```python
from build123d import *

# Parameters (mm, degrees)
SKETCH1_W           = 66.5
SKETCH1_H           = 36
SKETCH1_W_2         = 60.5
SKETCH1_H_2         = 30
BOSS_EXTRUDE1_DEPTH = 71
SKETCH1_3_W         = 66.5
SKETCH1_3_H         = 36
SKETCH1_3_W_2       = 60.5
SKETCH1_3_H_2       = 30
BOSS_EXTRUDE2_DEPTH = 3
CUT_EXTRUDE1_REACH  = 88.27
SKETCH2_W           = 15
SKETCH2_H           = 10
SKETCH4_W           = 1
SKETCH4_H           = 2
BOSS_EXTRUDE4_DEPTH = 15
CHAMFER1_SIZE       = 1
CUT_EXTRUDE2_DEPTH  = 1


with BuildPart() as part:
    # Sketch1 → Boss-Extrude1 (new body)
    with BuildSketch(Plane(origin=(0, 0, 0), x_dir=(1, 0, 0), z_dir=(0, 1, 0))):
        Rectangle(SKETCH1_W, SKETCH1_H)
        Rectangle(SKETCH1_W_2, SKETCH1_H_2, mode=Mode.SUBTRACT)
    extrude(amount=BOSS_EXTRUDE1_DEPTH)

    # Sketch1<3> → Boss-Extrude2 (add)
    with BuildSketch(Plane(origin=(0, 0, 0), x_dir=(1, 0, 0), z_dir=(0, 1, 0))):
        Rectangle(SKETCH1_3_W, SKETCH1_3_H)
        Rectangle(SKETCH1_3_W_2, SKETCH1_3_H_2, mode=Mode.SUBTRACT)
        Rectangle(SKETCH1_3_W_2, SKETCH1_3_H_2)
    extrude(amount=-BOSS_EXTRUDE2_DEPTH)

    # Sketch2 → Cut-Extrude1 (cut, up to next)
    with BuildSketch(Plane.XY.offset(18), mode=Mode.PRIVATE) as cut_extrude1_sk1:
        with Locations((0, 34)):
            Rectangle(SKETCH2_W, SKETCH2_H)
    cut_extrude1_tool1 = extrude(cut_extrude1_sk1.sketch, amount=-CUT_EXTRUDE1_REACH, mode=Mode.PRIVATE) & part.part
    add(cut_extrude1_tool1.solids().sort_by_distance((0, 34, 18))[0], mode=Mode.SUBTRACT)

    # Sketch4 → Boss-Extrude4 (add)
    with BuildSketch(Plane.ZY.offset(-7.5)):
        with Locations((14.5, 28)):
            Rectangle(SKETCH4_W, SKETCH4_H)
    extrude(amount=BOSS_EXTRUDE4_DEPTH)

    # Chamfer1
    chamfer1_edges = [part.edges().sort_by_distance(p)[0] for p in [
        (0, 29, 14),
    ]]
    chamfer(chamfer1_edges, length=CHAMFER1_SIZE)

    # Sketch5 → Cut-Extrude2 (cut)
    with BuildSketch(Plane(origin=(0, 0, -18), x_dir=(-1, 0, 0), z_dir=(0, 0, -1))):
        with BuildLine():
            Line((-2.638888889, 38.722222222), (-2.638888889, 39))
            Line((-2.638888889, 39), (2.5, 39))
            Line((2.5, 39), (2.5, 38.722222222))
            Line((2.5, 38.722222222), (2.172309028, 38.722222222))
            add(Edge.make_bspline(
                [(2.172309028, 38.722222222), (2.104184293, 38.720949678), (1.974513104, 38.718527469), (1.790231692, 38.689739833), (1.625736646, 38.644148981), (1.528628421, 38.595662221), (1.482204861, 38.572482639)],
                knots=[0, 0, 0, 0, 1.144467932, 2.17842344, 3.129177061, 4, 4, 4, 4], degree=3))
            add(Edge.make_bspline(
                [(1.482204861, 38.572482639), (1.451706337, 38.554084379), (1.390014843, 38.516868933), (1.310783803, 38.438036518), (1.243641581, 38.341940776), (1.209171954, 38.269240619), (1.19140625, 38.231770833)],
                knots=[0, 0, 0, 0, 0.93343552, 1.888125192, 2.911536119, 4, 4, 4, 4], degree=3))
            add(Edge.make_bspline(
                [(1.19140625, 38.231770833), (1.184350586, 38.214575185), (1.16854678, 38.176059078), (1.15557603, 38.106048651), (1.139091299, 38.020392262), (1.129876754, 37.915742203), (1.121221924, 37.794954741), (1.114101268, 37.656759716), (1.113522404, 37.501150705), (1.111942587, 37.391201064), (1.111111111, 37.333333333)],
                knots=[0, 0, 0, 0, 0.491143652, 1.100100526, 1.878201893, 2.802922625, 3.87869145, 5.087223688, 6.466973141, 8, 8, 8, 8], degree=3))
            Line((1.111111111, 37.333333333), (1.111111111, 30.666666667))
            add(Edge.make_bspline(
                [(1.111111111, 30.666666667), (1.111939588, 30.608075204), (1.113524957, 30.495954931), (1.114136618, 30.336734675), (1.121108982, 30.194912102), (1.130079845, 30.070534861), (1.138829557, 29.962956044), (1.156182735, 29.873070769), (1.16828298, 29.799419433), (1.195529243, 29.72563882), (1.240143315, 29.646586055), (1.312990851, 29.562040058), (1.405657276, 29.483796342), (1.517159605, 29.411555124), (1.650210211, 29.350190049), (1.805638269, 29.308289334), (1.981882259, 29.281860539), (2.106374028, 29.279191428), (2.172309028, 29.277777778)],
                knots=[0, 0, 0, 0, 1.353804055, 2.590631371, 3.678090953, 4.633038001, 5.472823534, 6.167945078, 6.748082955, 7.192141313, 7.977799851, 8.831603391, 9.756085287, 10.771283584, 11.893005217, 13.125761034, 14.477707027, 16, 16, 16, 16], degree=3))
            Line((2.172309028, 29.277777778), (2.5, 29.277777778))
            Line((2.5, 29.277777778), (2.5, 29))
            Line((2.5, 29), (-2.638888889, 29))
            Line((-2.638888889, 29), (-2.638888889, 29.277777778))
            Line((-2.638888889, 29.277777778), (-2.313368056, 29.277777778))
            add(Edge.make_bspline(
                [(-2.313368056, 29.277777778), (-2.245251066, 29.279076928), (-2.115594618, 29.281549779), (-1.931900868, 29.309888715), (-1.76838513, 29.356309608), (-1.671870984, 29.404385876), (-1.625434028, 29.427517361)],
                knots=[0, 0, 0, 0, 1.147815573, 2.184795468, 3.126629849, 4, 4, 4, 4], degree=3))
            add(Edge.make_bspline(
                [(-1.625434028, 29.427517361), (-1.594905814, 29.445892719), (-1.533154265, 29.483061837), (-1.454093177, 29.562557374), (-1.38462361, 29.657817078), (-1.348756572, 29.730709883), (-1.330295139, 29.768229167)],
                knots=[0, 0, 0, 0, 0.928829741, 1.878808762, 2.908183361, 4, 4, 4, 4], degree=3))
            add(Edge.make_bspline(
                [(-1.330295139, 29.768229167), (-1.323206914, 29.785418433), (-1.307060225, 29.82457489), (-1.295055162, 29.894793912), (-1.277647574, 29.980267632), (-1.268863248, 30.084275321), (-1.26000169, 30.205758881), (-1.253094282, 30.343969196), (-1.252369885, 30.49957111), (-1.250820734, 30.60879845), (-1.25, 30.666666667)],
                knots=[0, 0, 0, 0, 0.491154816, 1.118830903, 1.878082211, 2.802823963, 3.878617243, 5.106317376, 6.466938293, 8, 8, 8, 8], degree=3))
            Line((-1.25, 30.666666667), (-1.25, 37.333333333))
            add(Edge.make_bspline(
                [(-1.25, 37.333333333), (-1.250801761, 37.391926604), (-1.252336008, 37.504050339), (-1.253291766, 37.663247301), (-1.259177025, 37.805200537), (-1.271446326, 37.928690427), (-1.280582203, 38.036174276), (-1.295723919, 38.125982088), (-1.312405424, 38.198748616), (-1.338621653, 38.273308229), (-1.385613233, 38.351596892), (-1.455981361, 38.439521903), (-1.551157589, 38.515346585), (-1.661938741, 38.588028597), (-1.793960563, 38.650297433), (-1.948902922, 38.691613339), (-2.12438389, 38.71806089), (-2.248154932, 38.720786263), (-2.313368056, 38.722222222)],
                knots=[0, 0, 0, 0, 1.355372936, 2.593633572, 3.682353377, 4.639723862, 5.46383559, 6.176261324, 6.744401302, 7.188974265, 7.998347102, 8.842429006, 9.78074911, 10.797123889, 11.904961153, 13.139145573, 14.492658294, 16, 16, 16, 16], degree=3))
            Line((-2.313368056, 38.722222222), (-2.638888889, 38.722222222))
        make_face()
    extrude(amount=-CUT_EXTRUDE2_DEPTH, mode=Mode.SUBTRACT)


solid = part.part
```
The listing builds one solid part. Answer for the finished solid, in the listing's coordinates (mm). A direction names the side the tool comes from. Give positions to 0.01 mm unless a question says otherwise; leave off trailing zeros. Order: outer loops, then holes, each group sorted by start corner. A loop starts at its lowest first (then second) coordinate and runs counter-clockwise, first axis right, second up. Notation, with made-up numbers: M -37.75,-30 L 4.25,-30 A17 cw 4.25,-20 Z; hole C -31,-15.5 d9. An arc over 180 degrees is marked long. Put each result on its own line as item: value. Start each with the question number.
Item 1: The part is cut by section D-D, the plane z = 1. Determine the outline of the cut face in (x, y), and give its area (4 significant figures).
Item 2: For a pull along Z with two mould halves and no side action, classify faces 6 (the face through (-8, 35, 18)), 7 (the face through (-33.25, 35, 0)), 8 (the face through (0, 43, 15)) as +Z half, -Z half, draft (parallel to the pull), parting line (faces both ways), or undercut.
Item 3: Which of the six approach directions +Z, -Z, +X, -X, +Y, -Y give full straight-line access (tool end or side, diameter ignored) to faces 1 (the face through (7.5, 34, 17)), 2 (the face through (-30.25, 35, 0)), 3 (the face through (0, 34, -17)), 4 (the face through (-8, 35, -18)), 5 (the face through (0, -3, 0))?
Item 4: The part is cut by section A-A, the plane y = 5.5. Determine the outline of the cut face in (x, z), and give its area (3 significant figures).
Item 5: The part is cut by section C-C, the plane y = 32. Determine the outline of the cut face in (x, z).
Item 6: A flat-ended cylindrical pin translates along its axis: P1, Ø12, axis at x = -15.5, z = -1, coming from the +Y side. Find the tip coordinate at first contact, or state that the pin passes through.
Item 7: The part is cut by section B-B, the plane x = -12. Determine the outline of the cut face in (y, z), and give its area (3 significant figures).
Item 8: Find the intervals of material crossed by line 1 along X through (y, z) = (11.5, -10); line 2 along Z through (x, y) = (-20, 60); line 3 along Y through (x, z) = (0, 2.5), in increasing order.
Answer key:
1. outline: M -33.25,-3 L 33.25,-3 L 33.25,71 L 30.25,71 L 30.25,0 L -30.25,0 L -30.25,71 L -33.25,71 Z
1. area: 625.5 mm²
2. face 6: +Z half
2. face 7: draft
2. face 8: undercut
3. face 1: +Z
3. face 2: +Y
3. face 3: -Z
3. face 4: -Z, +X, -X, +Y, -Y
3. face 5: +Z, -Z, +X, -X, -Y
4. outline: M -33.25,-18 L 33.25,-18 L 33.25,18 L -33.25,18 Z; hole M -30.25,-15 L 30.25,-15 L 30.25,15 L -30.25,15 Z
4. area: 579 mm²
5. outline: M -33.25,-18 L -1.11,-18 L -1.11,-17 L 1.25,-17 L 1.25,-18 L 33.25,-18 L 33.25,18 L 7.5,18 L 7.5,15 L 30.25,15 L 30.25,-15 L -30.25,-15 L -30.25,15 L -7.5,15 L -7.5,18 L -33.25,18 Z
6. P1: stops at y = 0
7. outline: M -3,-18 L 71,-18 L 71,-15 L 0,-15 L 0,15 L 71,15 L 71,18 L -3,18 Z
7. area: 534 mm²
8. line 1: x = -33.25 to -30.25, 30.25 to 33.25
8. line 2: z = -18 to -15, 15 to 18
8. line 3: y = -3 to 0
